from build123d import *

# Parameters (mm, degrees)
SKETCH1_R           = 2
BOSS_EXTRUDE1_DEPTH = 4.5


with BuildPart() as part:
    # Sketch1 → Boss-Extrude1 (new body)
    with BuildSketch(Plane(origin=(0, 0, 0), x_dir=(0, 0, -1), z_dir=(1, 0, 0))):
        Polygon((-30.84603871, 0), (-40.84603871, 0), (-45.84603871, 5), (-40.84603871, 5), (-40.84603871, 15), (-60.84603871, 15), (-60.84603871, -15), (274.65396129, -15), (274.65396129, 5), (284.65396129, 5), (284.65396129, 0), (289.65396129, 5), (289.65396129, 15), (274.65396129, 15), (-30.84603871, 15), align=None)
        with Locations((-48.84603871, -3)):
            Circle(SKETCH1_R, mode=Mode.SUBTRACT)
        with Locations((264.65396129, -9)):
            Circle(SKETCH1_R, mode=Mode.SUBTRACT)
    extrude(amount=BOSS_EXTRUDE1_DEPTH)


solid = part.part
The listing builds one solid part. Answer for the finished solid, in the listing's coordinates (mm). Round coordinates to 2 decimals unless told otherwise and drop trailing zeros. Loops run counter-clockwise (first coordinate to the right, second up) from the corner with the lowest first, then second, coordinate; pieces in that order, holes last. Notation, with made-up numbers: M 83.25,3 L 91.25,3 A13 ccw 91.25,14 Z; hole C -15,-10 d1. An arc over 180 degrees is marked long. Return JSON: item names as keys, results as strings.
Q1. Each of these flat-tipped pins is pushed along its axis until it touches: pin 1 Ø2 at (x, z) = (2.5, 38) entering from +Y; pin 2 Ø3.5 at (y, z) = (-3, 48.85) entering from -X; pin 3 Ø2 at (x, y) = (3, -2) entering from -Z. Where does it stop, or does it pass through?
Results list:
{"pin 1": "stops at y = 0", "pin 2": "passes through", "pin 3": "stops at z = -274.65"}
Q2. Find section B-B, the plane x = 3.5. Determine the outline of the cut face in (y, z), plus the area to 3 significant figures.
Results list:
{"outline": "M -15,-274.65 L 5,-274.65 L 5,-284.65 L 0,-284.65 L 5,-289.65 L 15,-289.65 L 15,30.85 L 0,30.85 L 0,40.85 L 5,45.85 L 5,40.85 L 15,40.85 L 15,60.85 L -15,60.85 Z; hole C -9,-264.65 d4; hole C -3,48.85 d4", "area": "10,000 mm2"}
Q3. Find the intervals of material crossed by line 1 along Z through (x, y) = (2.45, 8.25); line 2 along Z through (x, y) = (2.2, -3.25), in increasing order. Write a range as from..to.
Results list:
{"line 1": "z = -289.65..30.85, 40.85..60.85", "line 2": "z = -274.65..46.86, 50.83..60.85"}
Q4. Find section A-A, the plane y = 11.5. Determine the outline of the cut face in (x, z).
Results list:
{"outline": "M 0,-289.65 L 4.5,-289.65 L 4.5,30.85 L 0,30.85 Z; M 0,40.85 L 4.5,40.85 L 4.5,60.85 L 0,60.85 Z"}
